Work out the finished part from the listing and answer in its coordinate system (mm). Round coordinates to 2 decimals unless told otherwise and drop trailing zeros. Loops run counter-clockwise (first coordinate to the right, second up) from the corner with the lowest first, then second, coordinate; pieces in that order, holes last. Notation, with made-up numbers: (34.25, -1.75) -> (46.25, -1.75) arc R15 ccw to (46.25, 15.25) -> close; hole circle Ø4 at (-14, 78.25). An arc over 180 degrees is marked (long way). Use one line per item in the form item = value.
```python
from build123d import *

# Parameters (mm, degrees)
SKETCH4_R          = 21
CUT_EXTRUDE1_DEPTH = 1.37
CUT_EXTRUDE1_DRAFT = -50
SKETCH5_W          = 2
SKETCH5_H          = 0.6


with BuildPart() as part:
    # Sketch3 → Revolve2 (revolve)
    with BuildSketch(Plane.XY, mode=Mode.PRIVATE) as revolve2_sk:
        with BuildLine():
            Line((-28, -2.8), (-28, -3.8))
            Line((-28, -3.8), (-21.291666667, -6.8))
            Line((-21.291666667, -6.8), (-19.589543983, -9.313904271))
            Line((-19.589543983, -9.313904271), (-31.8, -3.853327667))
            Line((-31.8, -3.853327667), (-31.8, 1.4))
            Line((-31.8, 1.4), (-29.8, 1.4))
            Line((-29.8, 1.4), (-29.8, -0.6))
            ThreePointArc((-29.8, -0.6), (-30.5, -2.1), (-29.8, -3.6))
            Line((-29.8, -3.6), (-29.8, -2.8))
            Line((-29.8, -2.8), (-28, -2.8))
        make_face()
    revolve(revolve2_sk.sketch.rotate(Axis((0, 0, 0), (0, 1, 0)), 270), axis=Axis((0, 0, 0), (0, 1, 0)))


with BuildPart() as cut_extrude1_tool:
    # Sketch4 → Cut-Extrude1 (with draft: the straight prism first)
    with BuildSketch(Plane(origin=(0, -9.313904271, 0), x_dir=(1, 0, 0), z_dir=(0, 1, 0))):
        Circle(SKETCH4_R)
    extrude(amount=CUT_EXTRUDE1_DEPTH)
    # Cut-Extrude1: the draft: its side faces are tilted about the plane it starts from
    cut_extrude1_sides = [cut_extrude1_tool.faces().sort_by_distance(p)[0] for p in [
        (-21, -8.628904271, 0),
    ]]
    draft(cut_extrude1_sides, Plane(origin=(0, -9.313904271, 0), x_dir=(1, 0, 0), z_dir=(0, 1, 0)), CUT_EXTRUDE1_DRAFT)


with BuildPart() as part_1:
    add(part.part)

    # Cut-Extrude1: cut by cut_extrude1_tool
    add(cut_extrude1_tool.part, mode=Mode.SUBTRACT)

    # Sketch5 → Cut-Revolve1 (revolve, cut)
    with BuildSketch(Plane.XY, mode=Mode.PRIVATE) as cut_revolve1_sk:
        with Locations((-30.8, 1.1)):
            Rectangle(SKETCH5_W, SKETCH5_H)
    revolve(cut_revolve1_sk.sketch.rotate(Axis((0, 0, 0), (0, 1, 0)), 270), axis=Axis((0, 0, 0), (0, 1, 0)), mode=Mode.SUBTRACT)

    # Sketch6 → Cut-Revolve2 (revolve, cut)
    with BuildSketch(Plane.XY, mode=Mode.PRIVATE) as cut_revolve2_sk:
        Polygon((-28, -3.8), (-29.8, -2.8), (-28, -2.8), align=None)
    revolve(cut_revolve2_sk.sketch.rotate(Axis((0, 0, 0), (0, 1, 0)), 90), axis=Axis((0, 0, 0), (0, 1, 0)), mode=Mode.SUBTRACT)

    # Sketch7 → Cut-Revolve3 (revolve, cut)
    with BuildSketch(Plane.XY, mode=Mode.PRIVATE) as cut_revolve3_sk:
        Polygon((-28, -3.8), (-21.291666667, -6.8), (-20.51714815, -7.943904271), (-29.8, -3.6), (-29.8, -2.8), align=None)
    revolve(cut_revolve3_sk.sketch.rotate(Axis((0, 0, 0), (0, 1, 0)), 90), axis=Axis((0, 0, 0), (0, 1, 0)), mode=Mode.SUBTRACT)


solid = part_1.part
```
(1) Find section D-D, the plane y = -2.5. Write down the section's boundary in (x, z), then the cut area to 3 significant figures.
Completed:
outline = circle Ø63.6 at (0, 0); hole circle Ø60.92 at (0, 0)
area = 262 mm2
(2) Consider L1, parallel to X at y = -0.2, z = 0; L2, parallel to X at y = 0, z = -22.5; L3, parallel to Z at x = -15, y = -3.5. Determine where each line is inside the solid, lowest interval first.
Completed:
L1 = -31.8 to -29.8, 29.8 to 31.8
L2 = -22.47 to -19.54, 19.54 to 22.47
L3 = -28.04 to -25.88, 25.88 to 28.04
(3) Find section C-C, the plane y = -6.5. Write down the section's boundary in (x, z), then the cut area to 3 significant figures.
Completed:
outline = circle Ø51.76 at (0, 0); hole circle Ø47.21 at (0, 0)
area = 354 mm2
(4) Given P1, Ø1.5, axis at x = -17, z = -22, coming from the +Y side; P2, Ø1, axis at x = 5, z = -20, coming from the +Y side; P3, Ø3, axis at x = 16, y = -4, coming from the +Z side, each flat-ended and moving along its own axis, determine where each tip first touches the part or whether it passes through.
Completed:
P1 = -4.18
P2 = -7.66
P3 = 28.3
(5) For a pull along X with two mould halves and no side action, classify faces 1 (the conical face through (-6.96, -7.71, -22.11)), 2 (the flat face through (-28.4, 0.8, 9.6)), 3 (the cylindrical face through (26.44, 0.09, -13.75)) as +X half, -X half, draft (parallel to the pull), parting line (faces both ways), or undercut.
Completed:
face_1 = parting line
face_2 = draft
face_3 = undercut
